```python
from build123d import *

# Parameters (mm, degrees)
F1_DEPTH = 18


# Not quite as in the source:
# - a feature names something its author has since deleted; it is built from what else it names


with BuildPart() as f1:
    # F0 (on Front) → F1 (new body)
    with BuildSketch(Plane.XZ):
        Polygon((0, 1000), (0, 0), (41, 0), (41, 125), (23, 125), (23, 250), (41, 250), (41, 375), (23, 375), (23, 500), (41, 500), (41, 625), (23, 625), (23, 750), (41, 750), (41, 875), (23, 875), (23, 1000), align=None)
    extrude(amount=F1_DEPTH)


solid = f1.part
```
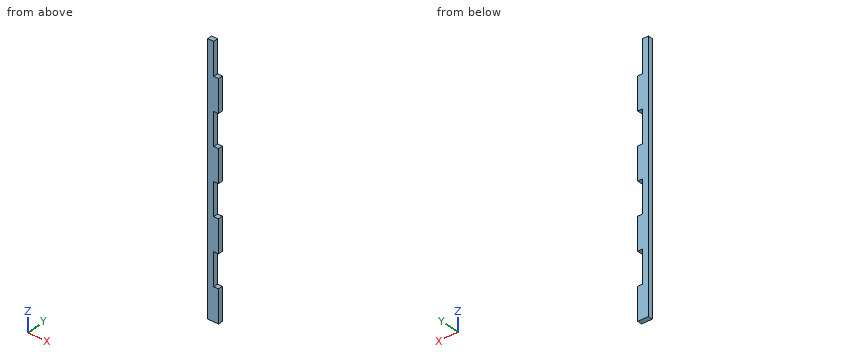
Can you work these out from the model? Positions are in its coordinate system, mm. Give positions to 0.01 mm unless a question says otherwise; leave off trailing zeros. Loops run counter-clockwise (first coordinate to the right, second up) from the corner with the lowest first, then second, coordinate; pieces in that order, holes last. Notation, with made-up numbers: M 70.25,43.25 L 86.25,43.25 A15 cw 86.25,61.25 Z; hole C 31.5,4.25 d11. An arc over 180 degrees is marked long. One line per question, with ' | ' between items. Start each with the question number.
Q1. If we section it at A-A (x = 32.5): Please give me the cut outline in (y, z), plus the area to 3 significant figures.
Q2. If we section it at B-B (y = -11.75): Please give me the cut outline in (x, z), plus the area to 3 significant figures.
Q3. If I drill on line 1 (Z direction, x = 36, y = -14.25); line 2 (X direction, y = -5.75, z = 648.5), over which ranges is the centre line in solid material (lowest first)? Write a range as from..to.
Q4. For pin 1 Ø9 at (y, z) = (-9, 942.5) entering from +X; pin 2 Ø1.5 at (x, z) = (7.5, 479.5) entering from +Y; pin 3 Ø9 at (x, y) = (32, -11) entering from +Z, each with a flat end and sliding along its axis, tell me the tip position at first contact or that it passes through.
Q5. If we section it at C-C (z = 938): Please give me the cut outline in (x, y), plus the area to 3 significant figures.
Computed:
1) outline: M -18,0 L 0,0 L 0,125 L -18,125 Z; M -18,250 L 0,250 L 0,375 L -18,375 Z; M -18,500 L 0,500 L 0,625 L -18,625 Z; M -18,750 L 0,750 L 0,875 L -18,875 Z | area: 9,000 mm²
2) outline: M 0,0 L 41,0 L 41,125 L 23,125 L 23,250 L 41,250 L 41,375 L 23,375 L 23,500 L 41,500 L 41,625 L 23,625 L 23,750 L 41,750 L 41,875 L 23,875 L 23,1000 L 0,1000 Z | area: 32,000 mm²
3) line 1: z = 0..125, 250..375, 500..625, 750..875 | line 2: x = 0..23
4) pin 1: stops at x = 23 | pin 2: stops at y = 0 | pin 3: stops at z = 875
5) outline: M 0,-18 L 23,-18 L 23,0 L 0,0 Z | area: 414 mm²
